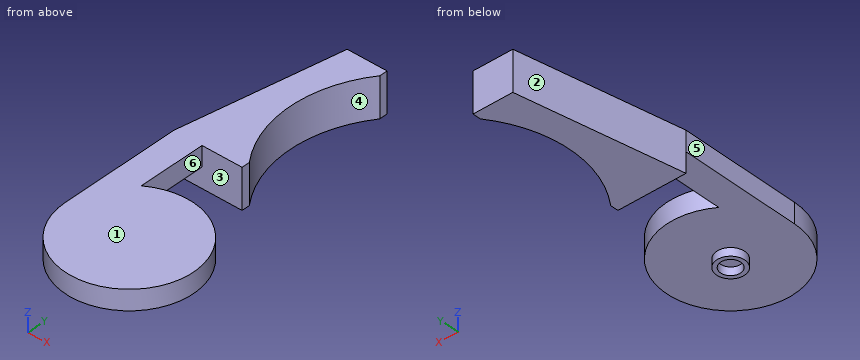
```python
from build123d import *

# Parameters (mm, degrees)
SKETCH1_R           = 20.32
BOSS_EXTRUDE1_DEPTH = 6.35
SKETCH2_R           = 4.445
SKETCH2_R_2         = 3.175
BOSS_EXTRUDE2_DEPTH = 2.54
SKETCH4_W           = 8.89
SKETCH4_H           = 38.1
BOSS_EXTRUDE3_DEPTH = 6.35
BOSS_EXTRUDE4_DEPTH = 12.7


with BuildPart() as part:
    # Sketch1 → Boss-Extrude1 (new body)
    with BuildSketch(Plane.XY):
        Circle(SKETCH1_R)
    extrude(amount=BOSS_EXTRUDE1_DEPTH)

    # Sketch2 → Boss-Extrude2 (add)
    with BuildSketch(Plane(origin=(0, 0, 0), x_dir=(-1, 0, 0), z_dir=(0, 0, -1))):
        with Locations(Location((0, 0, 0), (0, 0, 180))):
            Circle(SKETCH2_R)
        Circle(SKETCH2_R_2, mode=Mode.SUBTRACT)
    extrude(amount=BOSS_EXTRUDE2_DEPTH)

    # Sketch4 → Boss-Extrude3 (add)
    with BuildSketch(Plane.XY.offset(6.35)):
        with Locations((-15.875, 19.05)):
            Rectangle(SKETCH4_W, SKETCH4_H)
    extrude(amount=-BOSS_EXTRUDE3_DEPTH)

    # Sketch5 → Boss-Extrude4 (add)
    with BuildSketch(Plane.XY.offset(6.35)):
        with BuildLine():
            Line((-20.32, 38.1), (-11.36258938, 88.9))
            Line((-11.36258938, 88.9), (1.27, 88.9))
            Line((1.27, 88.9), (1.27, 86.36))
            ThreePointArc((1.27, 86.36), (-6.35, 63.5), (1.27, 40.64))
            Line((1.27, 40.64), (1.27, 38.1))
            Line((1.27, 38.1), (-11.43, 38.1))
            Line((-11.43, 38.1), (-20.32, 38.1))
        make_face()
    extrude(amount=-BOSS_EXTRUDE4_DEPTH)


solid = part.part
```
Verification items for the finished model (mm, model axes). Face numbers are marked on the shaded views. A direction names the side the tool comes from. Coordinates: 2 decimals unless noted, no trailing zeros. Loops run counter-clockwise (first coordinate to the right, second up) from the corner with the lowest first, then second, coordinate; pieces in that order, holes last. Notation, with made-up numbers: (-35.5, -6.75) - (-27.5, -6.75) arc R10 cw to (-27.5, 2.25) - close; hole circle Ø3 at (55.5, 43.25). An arc over 180 degrees is marked (long way). Return JSON: item names as keys, results as strings.
1. Go/stop test with flat-tipped pins: pin 1 (7 mm diameter, centred on y = 22, z = 4, fed in from +X); pin 2 (8.5 mm diameter, centred on x = 0, y = 0, fed in from -Z); pin 3 (0.8 mm diameter, centred on y = 40, z = 0.5, fed in from +X). Record where each tip stops, or that it passes through.
Established:
{"pin 1": "stops at x = 8.41", "pin 2": "stops at z = -2.54", "pin 3": "stops at x = 1.27"}
2. Section check B-B, the plane x = 0. Record the boundary of the cut face in (y, z) (3 decimals), then the cut area to 3 significant figures.
Established:
{"outline": "(-20.32, 0) - (-4.445, 0) - (-4.445, -2.54) - (-3.175, -2.54) - (-3.175, 0) - (3.175, 0) - (3.175, -2.54) - (4.445, -2.54) - (4.445, 0) - (20.32, 0) - (20.32, 6.35) - (-20.32, 6.35) - close; (38.1, -6.35) - (42.439, -6.35) - (42.439, 6.35) - (38.1, 6.35) - close; (84.561, -6.35) - (88.9, -6.35) - (88.9, 6.35) - (84.561, 6.35) - close", "area": "375 mm2"}
3. Section check A-A, the plane z = -1. Record the boundary of the cut face in (x, y) (3 decimals), then the cut area to 3 significant figures.
Established:
{"outline": "(-20.32, 38.1) - (1.27, 38.1) - (1.27, 40.64) arc R38.1 cw to (1.27, 86.36) - (1.27, 88.9) - (-11.363, 88.9) - close; circle Ø8.89 at (0, 0); hole circle Ø6.35 at (0, 0)", "area": "662 mm2"}
4. Section check D-D, the plane x = -15.5. Record the boundary of the cut face in (y, z), then the cut area to 3 significant figures.
Established:
{"outline": "(-13.14, 0) - (38.1, 0) - (38.1, -6.35) - (65.44, -6.35) - (65.44, 6.35) - (-13.14, 6.35) - close", "area": "673 mm2"}
5. Mould release check, pull along Y, two halves, no side actions. Record for the marked faces 1, 2, 3 and 4: +Y half, -Y half, draft (parallel to the pull), parting line (faces both ways), or undercut.
Established:
{"face 1": "draft", "face 2": "+Y half", "face 3": "undercut", "face 4": "undercut"}
6. Thickness scan on L1, parallel to Y at x = 0, z = -1.15 (3 decimals); L2, parallel to Z at x = -17, y = 22; L3, parallel to Y at x = 0.5, z = 1. Record the ranges inside material, lowest first.
Established:
{"L1": "y = -4.445 to -3.175, 3.175 to 4.445, 38.1 to 42.439, 84.561 to 88.9", "L2": "z = 0 to 6.35", "L3": "y = -20.31 to 20.31, 38.1 to 41.7, 85.3 to 88.9"}
7. Tool access check on the marked faces 5 and 6. Record the directions out of +Z, -Z, +X, -X, +Y, -Y that give a thin tool (end or side, any length) a straight path to the whole face; none if there is none.
Established:
{"face 5": "+Z, -Z, -X, +Y, -Y", "face 6": "+Z, -Z"}
8. Section check C-C, the plane y = 18.5. Record the boundary of the cut face in (x, z), then the cut area to 3 significant figures.
Established:
{"outline": "(-20.32, 0) - (-11.43, 0) - (-11.43, 6.35) - (-20.32, 6.35) - close; (-8.41, 0) - (8.41, 0) - (8.41, 6.35) - (-8.41, 6.35) - close", "area": "163 mm2"}
